```python
from build123d import *

# Parameters (mm, degrees)
SKETCH_W        = 44
SKETCH_H        = 42.000069
PAD_DEPTH       = 44
SKETCH001_W     = 39
SKETCH001_H     = 38.000069
POCKET_DEPTH    = 39
POCKET001_DEPTH = 42.001069
SKETCH003_R     = 1.5
SKETCH003_R_2   = 12
POCKET002_DEPTH = 44.001
SKETCH004_R     = 3
POCKET003_DEPTH = 5.001


with BuildPart() as part:
    # Sketch → Pad (new body)
    with BuildSketch(Plane.YZ):
        with Locations((22, 21.000034)):
            Rectangle(SKETCH_W, SKETCH_H)
    extrude(amount=PAD_DEPTH)

    # Sketch001 (on Face6 of Pad) → Pocket (cut)
    with BuildSketch(Plane.YZ.offset(44)):
        with Locations((24.5, 21.000034)):
            Rectangle(SKETCH001_W, SKETCH001_H)
    extrude(amount=-POCKET_DEPTH, mode=Mode.SUBTRACT)

    # Sketch002 (on Face6 of Pocket) → Pocket001 (cut, through all)
    with BuildSketch(Plane(origin=(0, 0, 42.000069), x_dir=(0, -1, 0), z_dir=(0, 0, 1))):
        Polygon((-44, 5), (-44, 44), (-5, 44), align=None)
    extrude(amount=-POCKET001_DEPTH, mode=Mode.SUBTRACT)

    # Sketch003 (on Face2 of Pocket001) → Pocket002 (cut, through all)
    with BuildSketch(Plane(origin=(0, 0, 0), x_dir=(0, 1, 0), z_dir=(-1, 0, 0))):
        with Locations((9, -5.500034)):
            Circle(SKETCH003_R)
        with Locations((40, -5.500034)):
            Circle(SKETCH003_R)
        with Locations((9, -36.500034)):
            Circle(SKETCH003_R)
        with Locations((40, -36.500034)):
            Circle(SKETCH003_R)
        with Locations((24.5, -21.000034)):
            Circle(SKETCH003_R_2)
    extrude(amount=-POCKET002_DEPTH, mode=Mode.SUBTRACT)

    # Sketch004 (on Face16 of Pocket002) → Pocket003 (cut, through all)
    with BuildSketch(Plane.ZX.offset(5)):
        with Locations((15, 36)):
            Circle(SKETCH004_R)
        with Locations((15, 13)):
            Circle(SKETCH004_R)
    extrude(amount=-POCKET003_DEPTH, mode=Mode.SUBTRACT)


solid = part.part
```
Read the model definition and answer for the solid it produces. Units are mm, in the model's axes. A direction names the side the tool comes from. Give positions to 0.01 mm unless a question says otherwise; leave off trailing zeros. Loops run counter-clockwise (first coordinate to the right, second up) from the corner with the lowest first, then second, coordinate; pieces in that order, holes last.
Item 1: Each of these flat-tipped pins is pushed along its axis until it touches: pin 1 Ø1 at (y, z) = (12, 18.5) entering from -X; pin 2 Ø4 at (y, z) = (9, 5.5) entering from +X; pin 3 Ø19 at (x, z) = (19.5, 29.5) entering from +Y. Where does it stop, or does it pass through?
Item 2: The mould has two halves that part along Z. Classify faces 3 (the flat face through (22, 0, 21)), 4 (the flat face through (17, 17, 42)), 5 (the cylindrical face through (2, 9, 38)), 6 (the flat face through (17, 17, 0)): released by +Z, released by -Z, zero draft, split by the parting line, or undercut.
Item 3: For faces 1 (the flat face through (5, 16, 30)), 2 (the cylindrical face through (2.5, 38.8, 6.4)), determine the directions among +Z, -Z, +X, -X, +Y, -Y from which every point of the face is accessible in a straight line to the end or side of a thin tool.
Item 4: The part is cut by section B-B (y = 24.5). Write down the section's boundary in (x, z), and give its area (3 significant figures).
Item 5: The part is cut by section C-C (y = 9). Write down the section's boundary in (x, z).
Item 6: The part is cut by section A-A (x = 13). Write down the section's boundary in (y, z).
Item 7: Find the intervals of material crossed by line 1 along Z through (x, y) = (1, 9); line 2 along X through (y, z) = (3.35, 15); line 3 along Z through (x, y) = (6, 32), in increasing order.
Item 8: The part is cut by section D-D (z = 34). Write down the section's boundary in (x, y), and give its area (3 significant figures).
Taken from the geometry:
1. pin 1: stops at x = 0
1. pin 2: stops at x = 5
1. pin 3: stops at y = 5
2. face 3: zero draft
2. face 4: released by +Z
2. face 5: undercut
2. face 6: released by -Z
3. face 1: +X, +Y
3. face 2: +X, -X
4. outline: (0, 0) - (24.5, 0) - (24.5, 2) - (5, 2) - (5, 9) - (0, 9) - close; (0, 33) - (5, 33) - (5, 40) - (24.5, 40) - (24.5, 42) - (0, 42) - close
4. area: 168 mm2
5. outline: (0, 0) - (40, 0) - (40, 2) - (5, 2) - (5, 4) - (0, 4) - close; (0, 7) - (5, 7) - (5, 35) - (0, 35) - close; (0, 38) - (5, 38) - (5, 40) - (40, 40) - (40, 42) - (0, 42) - close
6. outline: (0, 0) - (36, 0) - (36, 2) - (5, 2) - (5, 12) - (0, 12) - close; (0, 18) - (5, 18) - (5, 40) - (36, 40) - (36, 42) - (0, 42) - close
7. line 1: z = 0 to 4, 7 to 35, 38 to 42
7. line 2: x = 0 to 10, 16 to 33, 39 to 44
7. line 3: z = 0 to 2, 40 to 42
8. outline: (0, 0) - (44, 0) - (44, 5) - (5, 5) - (5, 44) - (0, 44) - close
8. area: 415 mm2
